Could you check a few things on this drawing? It's one solid part, dimensions in mm from its lowest x, y, z. A direction names the side the tool comes from. Give positions to 0.01 mm unless a question says otherwise; leave off trailing zeros. Order: outer loops, then holes, each group sorted by start corner. A loop starts at its lowest first (then second) coordinate and runs counter-clockwise, first axis right, second up. Notation, with made-up numbers: (20.5, 59) -> (48.5, 59) arc R31 ccw to (48.5, 97) -> close; hole circle Ø11 at (2.25, 45). An arc over 180 degrees is marked (long way). Answer as CSV lines item,"result".
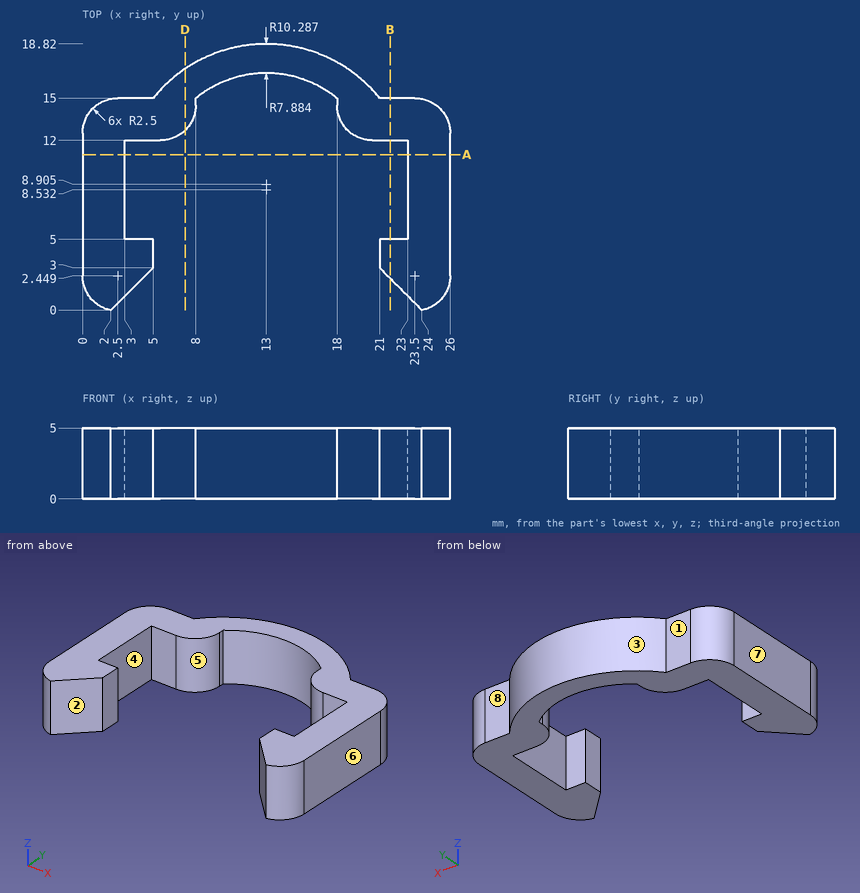
Item 1: Imagine slicing it at D-D, the plane x = 7.25. Please give me the cut outline in (y, z) (1 decimal).
Numbers:
outline,"(12.7, 0) -> (17.1, 0) -> (17.1, 5) -> (12.7, 5) -> close"
Item 2: Imagine slicing it at A-A, the plane y = 11. Please give me the cut outline in (x, z).
Numbers:
outline,"(0, 0) -> (3, 0) -> (3, 5) -> (0, 5) -> close; (23, 0) -> (26, 0) -> (26, 5) -> (23, 5) -> close"
Item 3: We'd pull the mould along X, two halves only. Please class the marked faces 5, 6, 7 and 8: released by +X, released by -X, zero draft, split by the parting line, or undercut.
Numbers:
face 5,"undercut"
face 6,"released by +X"
face 7,"released by -X"
face 8,"zero draft"
Item 4: For the marked faces 1, 2, 3 and 4, which set-ups out of +Z, -Z, +X, -X, +Y, -Y let a thin tool reach every point of the face, with its end or its side?
Numbers:
face 1,"+Z, -Z, -X, +Y"
face 2,"+Z, -Z, -Y"
face 3,"+Z, -Z, +Y"
face 4,"+Z, -Z"
Item 5: Please list where these lines run through material, in increasing order: line 1 along X through (y, z) = (9, 3.3); line 2 along Y through (x, z) = (21.5, 1); line 3 along X through (y, z) = (3.25, 4.8).
Numbers:
line 1,"x = 0 to 3, 23 to 26"
line 2,"y = 2.5 to 5, 12 to 15"
line 3,"x = 0 to 5, 21 to 26"
Item 6: For pin 1 (1.2 mm diameter, centred on x = 22.5, z = 2.5, fed in from -Y); pin 2 (0.6 mm diameter, centred on x = 22, z = 3.5, fed in from +Y); pin 3 (3 mm diameter, centred on x = 4.5, z = 2.5, fed in from -Y), each with a flat end and sliding along its axis, tell me the tip position at first contact or that it passes through.
Numbers:
pin 1,"stops at y = 0.9"
pin 2,"stops at y = 15"
pin 3,"stops at y = 1"
Item 7: Imagine slicing it at B-B, the plane x = 21.75. Please give me the cut outline in (y, z).
Numbers:
outline,"(2.25, 0) -> (5, 0) -> (5, 5) -> (2.25, 5) -> close; (12, 0) -> (15, 0) -> (15, 5) -> (12, 5) -> close"
